Here's how the part is built. I have some questions about the finished solid (model axes, mm). A direction names the side the tool comes from. Give positions to 0.01 mm unless a question says otherwise; leave off trailing zeros. Loops run counter-clockwise (first coordinate to the right, second up) from the corner with the lowest first, then second, coordinate; pieces in that order, holes last.
Q1. Suppose I cut it at C-C (x = 39). List the corners of the cut face in (y, z) for me, and give its area (3 significant figures).
Q2. Suppose I cut it at A-A (z = 40). List the corners of the cut face in (x, y) for me, and give its area (3 significant figures).
Q3. Suppose I cut it at B-B (y = 25). List the corners of the cut face in (x, z) for me.
Q4. Suppose I cut it at D-D (x = 22.5). List the corners of the cut face in (y, z) for me.
Q5. I need wall thicknesses on probe 1 along X at (y, z) = (11, 22); probe 2 along X at (y, z) = (4.5, 12.5); probe 3 along X at (y, z) = (13, 65). Which ranges of each line are inside material? Lowest first, please.
Q6. Thinking about a two-plate mould opening in X: for faces 4 (the face through (38, 0, 27)), 5 (the face through (100, 25, 10)), 6 (the face through (35, 24.7, 29.6)), 7 (the face through (0, 25, 27)), which applies, pulls with the +X half, pulls with the -X half, needs draft (parallel to the pull), parting line crosses it, or undercut?
Q7. I'm going to push flat-ended pins straight in: P1, Ø12.5, axis at x = 26.5, y = 15, coming from the -Z side; P2, Ø1, axis at y = 36.5, z = 39.5, coming from the +X side. Where does each tip first touch, or does it pass through?
Q8. For faces 1 (the face through (72, 25, 20)), 2 (the face through (17, 19, 60)), 3 (the face through (67, 25, 0)), which set-ups out of +Z, -Z, +X, -X, +Y, -Y let a thin tool reach every point of the face, with its end or its side?
```python
from build123d import *

# Parameters (mm, degrees)
F0_W     = 100
F0_H     = 50
F1_DEPTH = 20
F2_W     = 45
F2_H     = 50
F3_DEPTH = 50
F4_W     = 25
F4_H     = 60
F5_DEPTH = 50.001
F6_R     = 10
F7_DEPTH = 100.001
F8_R     = 7.5
F9_DEPTH = 10
F10_SIZE = 1
F11_R    = 1


with BuildPart() as f1:
    # F0 (on Top) → F1 (new body)
    with BuildSketch(Plane.XY):
        with Locations((50, 25)):
            Rectangle(F0_W, F0_H)
    extrude(amount=F1_DEPTH)

    # F2 (on face) → F3 (join)
    with BuildSketch(Plane.XY.offset(20)):
        with Locations((22.5, 25)):
            Rectangle(F2_W, F2_H)
    extrude(amount=F3_DEPTH)

    # F4 (on face) → F5 (cut, through all)
    with BuildSketch(Plane.XZ):
        with Locations((22.5, 30)):
            Rectangle(F4_W, F4_H)
    extrude(amount=-F5_DEPTH, mode=Mode.SUBTRACT)

    # F6 (on face) → F7 (cut, through all)
    with BuildSketch(Plane(origin=(0, 0, 0), x_dir=(0, -1, 0), z_dir=(-1, 0, 0))):
        with Locations((-25, 40)):
            Circle(F6_R)
    extrude(amount=-F7_DEPTH, mode=Mode.SUBTRACT)

    # F8 (on face) → F9 (cut, through all)
    with BuildSketch(Plane.XY.offset(70)):
        with Locations((22.5, 25)):
            Circle(F8_R)
    extrude(amount=-F9_DEPTH, mode=Mode.SUBTRACT)

    # F10
    f10_edges = [f1.edges().sort_by_distance(p)[0] for p in [
        (5, 0, 0),
        (0, 0, 35),
        (45, 0, 45),
        (22.5, 0, 70),
        (10, 0, 30),
        (22.5, 0, 60),
        (35, 0, 30),
        (67.5, 0, 0),
        (72.5, 0, 20),
        (100, 0, 10),
    ]]
    chamfer(f10_edges, length=F10_SIZE)

    # F11
    f11_edges = [f1.edges().sort_by_distance(p)[0] for p in [
        (0, 50, 35),
        (22.5, 50, 70),
        (45, 50, 45),
        (72.5, 50, 20),
        (100, 50, 10),
        (67.5, 50, 0),
        (35, 50, 30),
        (22.5, 50, 60),
        (10, 50, 30),
        (5, 50, 0),
    ]]
    fillet(f11_edges, radius=F11_R)


solid = f1.part
```
Solutions:
1. outline: (0, 1) - (1, 0) - (49, 0) arc R1 ccw to (50, 1) - (50, 69) arc R1 ccw to (49, 70) - (1, 70) - (0, 69) - close; hole circle Ø20 at (25, 40)
1. area: 3,180 mm2
2. outline: (0, 1) - (1, 0) - (9, 0) - (10, 1) - (10, 15) - (0, 15) - close; (0, 35) - (10, 35) - (10, 49) arc R1 ccw to (9, 50) - (1, 50) arc R1 ccw to (0, 49) - close; (35, 1) - (36, 0) - (44, 0) - (45, 1) - (45, 15) - (35, 15) - close; (35, 35) - (45, 35) - (45, 49) arc R1 ccw to (44, 50) - (36, 50) arc R1 ccw to (35, 49) - close
2. area: 597 mm2
3. outline: (0, 0) - (10, 0) - (10, 30) - (0, 30) - close; (0, 50) - (10, 50) - (10, 60) - (15, 60) - (15, 70) - (0, 70) - close; (30, 60) - (35, 60) - (35, 50) - (45, 50) - (45, 70) - (30, 70) - close; (35, 0) - (100, 0) - (100, 20) - (45, 20) - (45, 30) - (35, 30) - close
4. outline: (0, 61) - (1, 60) - (17.5, 60) - (17.5, 70) - (1, 70) - (0, 69) - close; (32.5, 60) - (49, 60) arc R1 ccw to (50, 61) - (50, 69) arc R1 ccw to (49, 70) - (32.5, 70) - close
5. probe 1: x = 0 to 10, 35 to 45
5. probe 2: x = 0 to 10, 35 to 100
5. probe 3: x = 0 to 45
6. face 4: needs draft
6. face 5: pulls with the +X half
6. face 6: undercut
6. face 7: pulls with the -X half
7. P1: stops at z = 60
7. P2: stops at x = 45
8. face 1: +Z, +X, +Y, -Y
8. face 2: -Z, +Y, -Y
8. face 3: -Z, +X, -X, +Y, -Y
